The listing builds one solid part. Answer for the finished solid, in the listing's coordinates (mm). A direction names the side the tool comes from. Give positions to 0.01 mm unless a question says otherwise; leave off trailing zeros. Loops run counter-clockwise (first coordinate to the right, second up) from the corner with the lowest first, then second, coordinate; pieces in that order, holes last. Notation, with made-up numbers: (72.25, 65) - (105.25, 65) arc R12 cw to (105.25, 75) - close; hole circle Ø9 at (48.25, 78). An arc over 180 degrees is marked (long way). Answer in a Markdown table with one row per item. Add a question column.
```python
from build123d import *

# Parameters (mm, degrees)
SKETCH1_R            = 20
BOSS_EXTRUDE4_DEPTH  = 11.938
SKETCH2_R            = 25
BOSS_EXTRUDE8_DEPTH  = 30
BOSS_EXTRUDE9_START  = 110.4
SKETCH7_R            = 25
BOSS_EXTRUDE9_DEPTH  = 110.4
SKETCH8_R            = 20
BOSS_EXTRUDE11_DEPTH = 11.9
BOSS_EXTRUDE12_START = -12.9
BOSS_EXTRUDE12_DEPTH = 12.9
SKETCH12_R           = 30
BOSS_EXTRUDE14_DEPTH = 10.5
BOSS_EXTRUDE15_START = 23
SKETCH14_R           = 25
BOSS_EXTRUDE15_DEPTH = 23
SKETCH15_R           = 5
BOSS_EXTRUDE17_DEPTH = 1.5
BOSS_EXTRUDE21_START = 5
SKETCH17_R           = 25
BOSS_EXTRUDE21_DEPTH = 5


with BuildPart() as part:
    # Sketch1 → Boss-Extrude4 (new body)
    with BuildSketch(Plane(origin=(0, 0, 0), x_dir=(1, 0, 0), z_dir=(0, 1, 0))):
        Circle(SKETCH1_R)
        with BuildLine():
            Line((-5.969, -19.088505416), (-5.969, -23.406505416))
            Line((-5.969, -23.406505416), (5.969, -23.406505416))
            Line((5.969, -23.406505416), (5.969, -19.088505416))
            ThreePointArc((5.969, -19.088505416), (0, -20), (-5.969, -19.088505416))
        make_face()
    extrude(amount=BOSS_EXTRUDE4_DEPTH)

    # Sketch2 → Boss-Extrude8 (add)
    with BuildSketch(Plane(origin=(0, 0, 0), x_dir=(1, 0, 0), z_dir=(0, 1, 0))):
        with Locations(Location((0, 0, 0), (0, 0, 270))):
            Circle(SKETCH2_R)
    extrude(amount=-BOSS_EXTRUDE8_DEPTH)

    # Sketch7 → Boss-Extrude9 (add)
    with BuildSketch(Plane(origin=(0, 11.938, 0), x_dir=(1, 0, 0), z_dir=(0, 1, 0)).offset(BOSS_EXTRUDE9_START)):
        with Locations(Location((0, 0, 0), (0, 0, 270))):
            Circle(SKETCH7_R)
    extrude(amount=-BOSS_EXTRUDE9_DEPTH)

    # Sketch8 → Boss-Extrude11 (add)
    with BuildSketch(Plane(origin=(0, 122.338, 0), x_dir=(1, 0, 0), z_dir=(0, 1, 0))):
        with Locations(Location((0, 0, 0), (0, 0, 90))):
            Circle(SKETCH8_R)
    extrude(amount=BOSS_EXTRUDE11_DEPTH)

    # Sketch9 → Boss-Extrude12 (add)
    with BuildSketch(Plane(origin=(0, 134.238, 0), x_dir=(1, 0, 0), z_dir=(0, 1, 0)).offset(BOSS_EXTRUDE12_START)):
        with BuildLine():
            Line((-5.95, 19.094436362), (-5.95, 23.394436362))
            Line((-5.95, 23.394436362), (5.95, 23.394436362))
            Line((5.95, 23.394436362), (5.95, 19.094436362))
            ThreePointArc((5.95, 19.094436362), (0, 20), (-5.95, 19.094436362))
        make_face()
    extrude(amount=BOSS_EXTRUDE12_DEPTH)

    # Sketch12 → Boss-Extrude14 (add)
    with BuildSketch(Plane(origin=(0, 134.238, 0), x_dir=(1, 0, 0), z_dir=(0, 1, 0))):
        with Locations(Location((0, 0, 0), (0, 0, 90))):
            Circle(SKETCH12_R)
    extrude(amount=BOSS_EXTRUDE14_DEPTH)

    # Sketch14 → Boss-Extrude15 (add)
    with BuildSketch(Plane(origin=(0, 144.738, 0), x_dir=(1, 0, 0), z_dir=(0, 1, 0)).offset(BOSS_EXTRUDE15_START)):
        with Locations(Location((0, 0, 0), (0, 0, 270))):
            Circle(SKETCH14_R)
    extrude(amount=-BOSS_EXTRUDE15_DEPTH)

    # Sketch15 → Boss-Extrude17 (add)
    with BuildSketch(Plane(origin=(0, 167.738, 0), x_dir=(1, 0, 0), z_dir=(0, 1, 0))):
        with Locations(Location((0, 8, 0), (0, 0, 270))):
            Circle(SKETCH15_R)
        with Locations(Location((0, -8, 0), (0, 0, 270))):
            Circle(SKETCH15_R)
    extrude(amount=BOSS_EXTRUDE17_DEPTH)

    # Sketch17 → Boss-Extrude21 (add)
    with BuildSketch(Plane(origin=(0, 169.238, 0), x_dir=(1, 0, 0), z_dir=(0, 1, 0)).offset(BOSS_EXTRUDE21_START)):
        with Locations(Location((0, 0, 0), (0, 0, 270))):
            Circle(SKETCH17_R)
    extrude(amount=-BOSS_EXTRUDE21_DEPTH)


solid = part.part
```
(1) Given pin 1 Ø8 at (x, y) = (9.5, 91.5) entering from -Z; pin 2 Ø1.5 at (y, z) = (19, 1) entering from +X; pin 3 Ø4.5 at (y, z) = (131, -22.5) entering from -X, each flat-ended and moving along its own axis, determine where each tip first touches the part or whether it passes through.
(2) A cutting plane is placed at A-A on z = 0. Determine the outline of the cut face in (x, y).
(3) A cutting plane is placed at D-D on y = 18.5. Determine the outline of the cut face in (x, z).
(4) A cutting plane is placed at B-B on x = -16.5. Determine the outline of the cut face in (y, z), plus the area to 3 significant figures.
(5) A tool of negligible diameter and unlimited length cuts with its end or side. For faces 4 (the face through (-7, 11.938, -19)), 5 (the face through (0, 128, -23.394)), 6 (the face through (7.509, 156.399, 23.846)), 7 (the face through (7.509, -14.79, 23.846)), from which of +Z, -Z, +X, -X, +Y, -Y can it reach the whole face along a straight path? Write none if from no direction.
(6) The mould has two halves that part along Z. Classify faces 1 (the face through (0, -30, 0)), 2 (the face through (1.5, 168.48, -3.23)), 3 (the face through (-0.795, 128.205, 19.984)): pulls with the +Z half, pulls with the -Z half, needs draft (parallel to the pull), parting line crosses it, or undercut.
(7) Find the intervals of material crossed by line 1 along Y through (x, z) = (14, 16.5); line 2 along Y through (x, z) = (4.5, 22.5); line 3 along Y through (x, z) = (-11.5, -11), in increasing order. Write a range as [from, to].
Evaluation:
| question | item | result |
|---|---|---|
| 1 | pin 1 | stops at z = -24.39 |
| 1 | pin 2 | stops at x = 25 |
| 1 | pin 3 | stops at x = -5.95 |
| 2 | outline | (-30, 134.24) - (-20, 134.24) - (-20, 122.34) - (-25, 122.34) - (-25, 11.94) - (-20, 11.94) - (-20, 0) - (-25, 0) - (-25, -30) - (25, -30) - (25, 0) - (20, 0) - (20, 11.94) - (25, 11.94) - (25, 122.34) - (20, 122.34) - (20, 134.24) - (30, 134.24) - (30, 144.74) - (25, 144.74) - (25, 167.74) - (-25, 167.74) - (-25, 144.74) - (-30, 144.74) - close; (-25, 169.24) - (25, 169.24) - (25, 174.24) - (-25, 174.24) - close |
| 3 | outline | circle Ø50 at (0, 0) |
| 4 | outline | (-30, -18.78) - (0, -18.78) - (0, -11.3) - (11.94, -11.3) - (11.94, -18.78) - (122.34, -18.78) - (122.34, -11.3) - (134.24, -11.3) - (134.24, -25.05) - (144.74, -25.05) - (144.74, -18.78) - (167.74, -18.78) - (167.74, 18.78) - (144.74, 18.78) - (144.74, 25.05) - (134.24, 25.05) - (134.24, 11.3) - (122.34, 11.3) - (122.34, 18.78) - (11.94, 18.78) - (11.94, 11.3) - (0, 11.3) - (0, 18.78) - (-30, 18.78) - close; (169.24, -18.78) - (174.24, -18.78) - (174.24, 18.78) - (169.24, 18.78) - close |
| 4 | area | 7,390 mm² |
| 5 | face 4 | none |
| 5 | face 5 | -Z, +X, -X |
| 5 | face 6 | +Y |
| 5 | face 7 | -Y |
| 6 | face 1 | needs draft |
| 6 | face 2 | undercut |
| 6 | face 3 | parting line crosses it |
| 7 | line 1 | y = [-30, 0], [11.94, 122.34], [134.24, 167.74], [169.24, 174.24] |
| 7 | line 2 | y = [-30, 122.34], [134.24, 167.74], [169.24, 174.24] |
| 7 | line 3 | y = [-30, 167.74], [169.24, 174.24] |
